from build123d import *

# Parameters (mm, degrees)
SKETCH3_W             = 9
SKETCH3_H             = 40
SKETCH3_R             = 1.5
BOSS_EXTRUDE5_DEPTH   = 2
BOSS_EXTRUDE5_2_DEPTH = 2
SKETCH5_W             = 46
SKETCH5_H             = 20
SKETCH5_R             = 1.5
BOSS_EXTRUDE7_DEPTH   = 2
SKETCH6_R             = 1.5
CUT_EXTRUDE1_DEPTH    = 10
SKETCH7_R             = 1.5
CUT_EXTRUDE2_DEPTH    = 10


with BuildPart() as part:
    # Sketch3 → Boss-Extrude5 (new body)
    with BuildSketch(Plane.XY):
        with Locations((-21.015808288, -14.438328765)):
            Rectangle(SKETCH3_W, SKETCH3_H)
        with Locations((-21.015808288, -29.438328765)):
            Circle(SKETCH3_R, mode=Mode.SUBTRACT)
        with Locations((-21.015808288, -6.938328765)):
            Circle(SKETCH3_R, mode=Mode.SUBTRACT)
    extrude(amount=BOSS_EXTRUDE5_DEPTH)



with BuildPart() as body_2:
    # Sketch3 → Boss-Extrude5 2 (new body)
    with BuildSketch(Plane.XY):
        with Locations((15.984191712, -14.438328765)):
            Rectangle(SKETCH3_W, SKETCH3_H)
        with Locations((15.984191712, -29.438328765)):
            Circle(SKETCH3_R, mode=Mode.SUBTRACT)
        with Locations((15.984191712, -6.938328765)):
            Circle(SKETCH3_R, mode=Mode.SUBTRACT)
    extrude(amount=BOSS_EXTRUDE5_2_DEPTH)


with BuildPart() as part_1:
    add(part.part)

    add(body_2.part)  # Boss-Extrude7 merges body 2
    # Sketch5 → Boss-Extrude7 (add)
    with BuildSketch(Plane(origin=(0, 4, 0), x_dir=(1, 0, 0), z_dir=(0, 1, 0))):
        with Locations((-2.515808288, 8)):
            Rectangle(SKETCH5_W, SKETCH5_H)
        with Locations(Location((-2.515808288, 13, 0), (0, 0, 270))):
            Circle(SKETCH5_R, mode=Mode.SUBTRACT)
    extrude(amount=BOSS_EXTRUDE7_DEPTH)

    # Sketch6 → Cut-Extrude1 (cut)
    with BuildSketch(Plane.XY.offset(2)):
        with Locations((15.834091702, -19.231630496)):
            Circle(SKETCH6_R)
    extrude(amount=-CUT_EXTRUDE1_DEPTH, mode=Mode.SUBTRACT)

    # Sketch7 → Cut-Extrude2 (cut)
    with BuildSketch(Plane.XY.offset(2)):
        with Locations((-21.127531315, -19.770890517)):
            Circle(SKETCH7_R)
    extrude(amount=-CUT_EXTRUDE2_DEPTH, mode=Mode.SUBTRACT)


solid = part_1.part
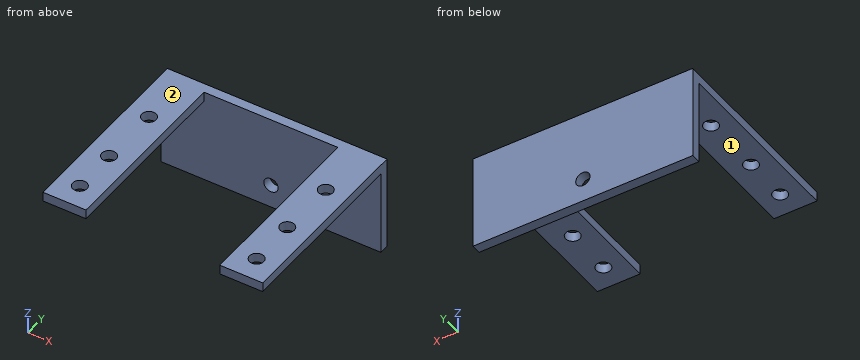
Can you work these out from the model? Positions are in its coordinate system, mm. Face numbers are marked on the shaded views. A direction names the side the tool comes from. Coordinates: 2 decimals unless noted, no trailing zeros. Write each loop counter-clockwise with the first axis right and the second up, starting at its lowest first coordinate (ties: lowest second). Pieces come first, ordered by that corner, then holes. Notation, with made-up numbers: (-16, 22.25) -> (35, 22.25) arc R15 cw to (35, 29.25) -> close; hole circle Ø11 at (-2.75, 73). An arc over 180 degrees is marked (long way). Answer as CSV lines item,"result".
1) If we section it at B-B on y = -13: Please give me the cut outline in (x, z).
Check result:
outline,"(-25.52, 0) -> (-16.52, 0) -> (-16.52, 2) -> (-25.52, 2) -> close; (11.48, 0) -> (20.48, 0) -> (20.48, 2) -> (11.48, 2) -> close"
2) If I drill on line 1 (X direction, y = -24, z = 0.75); line 2 (Y direction, x = -7, z = -13); line 3 (Z direction, x = -19.5, y = -1.5), over which ranges is the centre line in solid material (lowest first)? Write a range as from..to.
Check result:
line 1,"-25.52..-16.52, 11.48..20.48"
line 2,"4..6"
line 3,"0..2"
3) On a 3-axis mill with a long thin cutter (end or side, diameter ignored), from which of +Z, -Z, +X, -X, +Y, -Y can I reach the whole of each face in a straight line? I mean the marked faces 1 and 2. Say none if no direction works.
Check result:
face 1,"-Z, +X, -X, -Y"
face 2,"+Z, +X, -X, +Y, -Y"
4) If we section it at A-A on z = -13: Please give me the cut outline in (x, y), then the cut area to 3 significant figures.
Check result:
outline,"(-25.52, 4) -> (-4.02, 4) -> (-4.02, 6) -> (-25.52, 6) -> close; (-1.02, 4) -> (20.48, 4) -> (20.48, 6) -> (-1.02, 6) -> close"
area,"86.0 mm²"
5) If we section it at C-C on x = -6: Please give me the cut outline in (y, z).
Check result:
outline,"(4, -18) -> (6, -18) -> (6, 2) -> (4, 2) -> close"
6) If we section it at D-D on z = -2.5: Please give me the cut outline in (x, y), then the cut area to 3 significant figures.
Check result:
outline,"(-25.52, 4) -> (20.48, 4) -> (20.48, 6) -> (-25.52, 6) -> close"
area,"92.0 mm²"
7) Will these pins go through, and if not, where does the flat tip stop? P1, Ø2.5, axis at x = -2.52, z = -13, coming from the -Y side; P2, Ø10, axis at x = -21, y = -13, coming from the -Z side.
Check result:
P1,"through"
P2,"z = 0"
